For this review, take the finished solid that the model builds, in its own axes (mm). Face numbers are marked on the shaded views. A direction names the side the tool comes from. Give positions to 0.01 mm unless a question says otherwise; leave off trailing zeros. Write each loop counter-clockwise with the first axis right and the second up, starting at its lowest first coordinate (ties: lowest second). Pieces come first, ordered by that corner, then holes. Notation, with made-up numbers: (87, 24) -> (118, 24) arc R26 cw to (118, 39) -> close; hole circle Ø4 at (67, 32). An arc over 180 degrees is marked (long way). Answer as CSV lines item,"result".
```python
from build123d import *

# Parameters (mm, degrees)
BOSS_EXTRUDE1_DEPTH = 7
CUT_EXTRUDE1_REACH  = 15.252
SKETCH2_R           = 1.25
CUT_EXTRUDE2_REACH  = 14.743


with BuildPart() as part:
    # Sketch1 → Boss-Extrude1 (new body)
    with BuildSketch(Plane.XY):
        Polygon((-10, -3.659090909), (-2, -3.659090909), (-2, 0), (2, 0), (2, -3.659090909), (10, -3.659090909), (10, -2.159090909), (3.5, -2.159090909), (3.5, 1.5), (-3.5, 1.5), (-3.5, -2.159090909), (-10, -2.159090909), align=None)
    extrude(amount=BOSS_EXTRUDE1_DEPTH)

    # Sketch2 → Cut-Extrude1 (cut, up to next)
    with BuildSketch(Plane.XZ.offset(3.659090909), mode=Mode.PRIVATE) as cut_extrude1_sk1:
        with Locations(Location((5.000786438, 3.8, 0), (0, 0, 270))):
            Circle(SKETCH2_R)
    cut_extrude1_tool1 = extrude(cut_extrude1_sk1.sketch, amount=-CUT_EXTRUDE1_REACH, mode=Mode.PRIVATE) & part.part
    cut_extrude1 = cut_extrude1_tool1.solids().sort_by_distance((5.000786, -3.659091, 3.8))[0]
    add(cut_extrude1, mode=Mode.SUBTRACT)

    # Mirror1: Cut-Extrude1 across plane
    add(cut_extrude1.mirror(Plane.ZY), mode=Mode.SUBTRACT)

    # Sketch3 → Cut-Extrude2 (cut, up to next)
    with BuildSketch(Plane.XZ, mode=Mode.PRIVATE) as cut_extrude2_sk1:
        Polygon((0.974278579, 3.5), (-0.974278579, 4.625), (-0.974278579, 2.375), align=None)
    cut_extrude2_tool1 = extrude(cut_extrude2_sk1.sketch, amount=-CUT_EXTRUDE2_REACH, mode=Mode.PRIVATE) & part.part
    add(cut_extrude2_tool1.solids().sort_by_distance((-0.32476, 0, 3.5))[0], mode=Mode.SUBTRACT)


solid = part.part
```
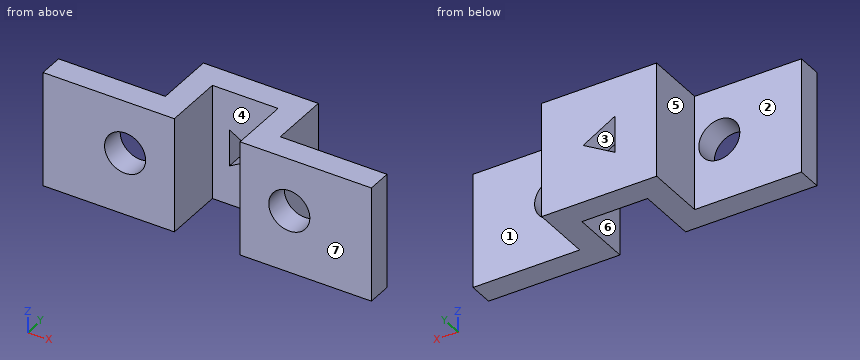
Q1. Add section C-C (y = 0.45). Write out the cut boundary in (x, z) (3 decimals).
Answer block:
outline,"(-3.5, 0) -> (3.5, 0) -> (3.5, 7) -> (-3.5, 7) -> close; hole (-0.974, 2.375) -> (0.974, 3.5) -> (-0.974, 4.625) -> close"
Q2. Add section A-A (y = -1.25). Write out the cut boundary in (x, z).
Answer block:
outline,"(-3.5, 0) -> (-2, 0) -> (-2, 7) -> (-3.5, 7) -> close; (2, 0) -> (3.5, 0) -> (3.5, 7) -> (2, 7) -> close"
Q3. Add section D-D (x = 5.25). Write out the cut boundary in (y, z), plus the area to 3 significant figures.
Answer block:
outline,"(-3.66, 0) -> (-2.16, 0) -> (-2.16, 2.58) -> (-3.66, 2.58) -> close; (-3.66, 5.02) -> (-2.16, 5.02) -> (-2.16, 7) -> (-3.66, 7) -> close"
area,"6.83 mm2"
Q4. For the marked faces 1, 2, 3 and 4, list the 3-axis set-ups (+Z, -Z, +X, -X, +Y, -Y) from which the entire face can be reached by the end or side of a thin tool; tool diameter is ignored.
Answer block:
face 1,"+Z, -Z, +X, +Y"
face 2,"+Z, -Z, -X, +Y"
face 3,"+Y, -Y"
face 4,"+Z, -Z, -Y"
Q5. Clearance check with flat-ended pins moving along their axes: pin 1 (3 mm diameter, centred on y = 0, z = 5.5, fed in from -X); pin 2 (3 mm diameter, centred on x = -5, z = 3.8, fed in from -Y); pin 3 (3 mm diameter, centred on x = -8, z = 2.5, fed in from +Y); pin 4 (2 mm diameter, centred on x = 5, z = 3.8, fed in from +Y). State where each tip first meets the part, or that it passes through.
Answer block:
pin 1,"stops at x = -3.5"
pin 2,"stops at y = -3.66"
pin 3,"stops at y = -2.16"
pin 4,"passes through"
Q6. Draft analysis for pull direction X (two halves, no side actions). For the marked faces 5, 6 and 7, state which applies: released by +X, released by -X, zero draft, split by the parting line, or undercut.
Answer block:
face 5,"released by -X"
face 6,"undercut"
face 7,"zero draft"
Q7. Add section B-B (z = 1.5). Write out the cut boundary in (x, y), plus the area to 3 significant figures.
Answer block:
outline,"(-10, -3.66) -> (-2, -3.66) -> (-2, 0) -> (2, 0) -> (2, -3.66) -> (10, -3.66) -> (10, -2.16) -> (3.5, -2.16) -> (3.5, 1.5) -> (-3.5, 1.5) -> (-3.5, -2.16) -> (-10, -2.16) -> close"
area,"41.0 mm2"
Q8. To check wall thickness, follow probe 1 along X at (y, z) = (-3.25, 3.75); probe 2 along X at (y, z) = (-0.4, 5). State the ranges of each line that lie inside material, in increasing order. Write a range as [from, to].
Answer block:
probe 1,"x = [-10, -6.25], [-3.75, -2], [2, 3.75], [6.25, 10]"
probe 2,"x = [-3.5, -2], [2, 3.5]"
